Could you check a few things on this model? Use its own coordinates, in mm. A direction names the side the tool comes from. Give positions to 0.01 mm unless a question says otherwise; leave off trailing zeros. Loops run counter-clockwise (first coordinate to the right, second up) from the corner with the lowest first, then second, coordinate; pieces in that order, holes last. Notation, with made-up numbers: M 25,52.5 L 33,52.5 A19 cw 33,79.5 Z; hole C -40,87 d7. An arc over 180 degrees is marked long. Use CSV: the item, a comma, the result in double quotes.
```python
from build123d import *

# Parameters (mm, degrees)
SKETCH1_W                       = 203.2
SKETCH1_H                       = 101.6
BOSS_EXTRUDE1_DEPTH             = 9.525
CUT_EXTRUDE1_DEPTH              = 93.98
CUT_EXTRUDE1_DEPTH_BACK         = 228.384092726
SKETCH2_W                       = 1.5875
SKETCH2_H                       = 50.8
CBORE_FOR_M5_SBHCS1_D           = 5.5
CBORE_FOR_M5_SBHCS1_CBORE_D     = 10.5
CBORE_FOR_M5_SBHCS1_CBORE_DEPTH = 2.75
M5_CLEARANCE_HOLE1_D            = 5.5


with BuildPart() as part:
    # Sketch1 → Boss-Extrude1 (new body)
    with BuildSketch(Plane.XY):
        with Locations((101.6, 50.8)):
            Rectangle(SKETCH1_W, SKETCH1_H)
    extrude(amount=BOSS_EXTRUDE1_DEPTH)

    # Sketch2 → Cut-Extrude1 (cut, two sides: drawn at the far end of the back side and taken through both)
    with BuildSketch(Plane(origin=(0, 0, 0), x_dir=(0, 0, -1), z_dir=(1, 0, 0)).offset(-CUT_EXTRUDE1_DEPTH_BACK)):
        with Locations((-0.79375, 50.8)):
            Rectangle(SKETCH2_W, SKETCH2_H)
    extrude(amount=CUT_EXTRUDE1_DEPTH + CUT_EXTRUDE1_DEPTH_BACK, mode=Mode.SUBTRACT)

    # CBORE for M5 SBHCS1 (through all)
    with Locations(Plane(origin=(0, 0, 0), x_dir=(-1, 0, 0), z_dir=(0, 0, -1))):
        with Locations((-190.5, 88.9), (-12.7, 88.9), (-12.7, 12.7), (-190.5, 12.7)):
            CounterBoreHole(CBORE_FOR_M5_SBHCS1_D / 2, CBORE_FOR_M5_SBHCS1_CBORE_D / 2, CBORE_FOR_M5_SBHCS1_CBORE_DEPTH)

    # M5 Clearance Hole1 (through all)
    with Locations(Plane.XY.offset(9.525)):
        with Locations((158.75, 50.8), (98.7552, 50.8)):
            Hole(M5_CLEARANCE_HOLE1_D / 2)


solid = part.part
```
1. I'm going to push flat-ended pins straight in: pin 1 Ø7 at (x, y) = (190.5, 12.7) entering from +Z (3 decimals); pin 2 Ø15 at (x, y) = (63, 59) entering from -Z; pin 3 Ø3 at (x, y) = (192, 10.5) entering from -Z; pin 4 Ø4.5 at (x, y) = (158.75, 50.8) entering from -Z. Where does each tip first touch, or does it pass through?
Outcome:
pin 1,"z = 9.525"
pin 2,"z = 1.59"
pin 3,"z = 2.75"
pin 4,"through"
2. I want a section at C-C, the plane x = 158.75. List the corners of the cut face in (y, z) for me (3 decimals).
Outcome:
outline,"M 0,0 L 48.05,0 L 48.05,9.525 L 0,9.525 Z; M 53.55,0 L 101.6,0 L 101.6,9.525 L 53.55,9.525 Z"
3. Which directions (+Z, -Z, +X, -X, +Y, -Y) give clear straight access to the entire face, cutting with the end or side of a thin tool? Please do faces 5 (the face through (10.28, 8.04, 1.36)), 6 (the face through (46, 50, 1.588)), 7 (the face through (12.104, 86.215, 6.185)).
Outcome:
face 5,"-Z"
face 6,"-Z, -X"
face 7,"+Z, -Z"
4. I want a section at B-B, the plane x = 190.5. List the corners of the cut face in (y, z) for me (3 decimals).
Outcome:
outline,"M 0,0 L 7.45,0 L 7.45,2.75 L 9.95,2.75 L 9.95,9.525 L 0,9.525 Z; M 15.45,2.75 L 17.95,2.75 L 17.95,0 L 83.65,0 L 83.65,2.75 L 86.15,2.75 L 86.15,9.525 L 15.45,9.525 Z; M 91.65,2.75 L 94.15,2.75 L 94.15,0 L 101.6,0 L 101.6,9.525 L 91.65,9.525 Z"
5. I want a section at D-D, the plane y = 50.8. List the corners of the cut face in (x, z) for me (1 decimal), then the cut area to 3 significant figures.
Outcome:
outline,"M 0,1.6 L 94,1.6 L 94,0 L 96,0 L 96,9.5 L 0,9.5 Z; M 101.5,0 L 156,0 L 156,9.5 L 101.5,9.5 Z; M 161.5,0 L 203.2,0 L 203.2,9.5 L 161.5,9.5 Z"
area,"1,680 mm2"
6. If we mould it in two halves opening along X, with no side actions, what happens to faces 1 (the face through (12.342, 15.427, 6.185)), 2 (the face through (193.12, 13.53, 6.18)), 3 (the face through (203.2, 50, 5)), 4 (the face through (0, 50, 5))? For each: +X half, -X half, draft (parallel to the pull), parting line (faces both ways), or undercut.
Outcome:
face 1,"undercut"
face 2,"undercut"
face 3,"+X half"
face 4,"-X half"
7. I want a section at A-A, the plane y = 12.7. List the corners of the cut face in (x, z) for me (3 decimals), then the cut area to 3 significant figures.
Outcome:
outline,"M 0,0 L 7.45,0 L 7.45,2.75 L 9.95,2.75 L 9.95,9.525 L 0,9.525 Z; M 15.45,2.75 L 17.95,2.75 L 17.95,0 L 185.25,0 L 185.25,2.75 L 187.75,2.75 L 187.75,9.525 L 15.45,9.525 Z; M 193.25,2.75 L 195.75,2.75 L 195.75,0 L 203.2,0 L 203.2,9.525 L 193.25,9.525 Z"
area,"1,800 mm2"
8. Please list where these lines run through material, in increasing order: line 1 (Y direction, x = 190.5, z = 1.55); line 2 (Y direction, x = 190.5, z = 7.75); line 3 (X direction, y = 89, z = 5.25).
Outcome:
line 1,"0 to 7.45, 17.95 to 83.65, 94.15 to 101.6"
line 2,"0 to 9.95, 15.45 to 86.15, 91.65 to 101.6"
line 3,"0 to 9.95, 15.45 to 187.75, 193.25 to 203.2"
